Solid Edge part; units mm, degrees
sketch "Sketch1" plane through (0, 0, 0) normal (0, -1, 0) x (1, 0, 0)
  line L0 (-60, 0) -> (-60, 9)
  line L1 (-60, 9) -> (-59, 10)
  line L2 (-59, 10) -> (164, 10)
  line L3 (164, 16) -> (164, 10)
  line L4 (176, 16) -> (164, 16)
  line L5 (176, 10) -> (176, 16)
  line L6 (194, 10) -> (176, 10)
  line L7 (194, 8) -> (194, 10)
  line L8 (224, 8) -> (194, 8)
  line L9 (224, 6) -> (224, 8)
  line L10 (239, 6) -> (224, 6)
  line L11 (239, 6) -> (240, 5)
  line L12 (240, 0) -> (240, 5)
revolve "RevolvedProtrusion1" add sketch "Sketch1" angle 360 about axis through (-60, 0, 0) along (1, 0, 0)
cosmetic_thread "Thread1"
cosmetic_thread "Thread2"
sketch "Sketch2" plane through (224, 0, 0) normal (1, 0, 0) x (0, 1, 0)
  line L0 (-2.5, 5.5) -> (2.5, 5.5)
  line L1 (2.5, 5.5) -> (2.5, 10.5)
  line L2 (2.5, 10.5) -> (-2.5, 10.5)
  line L3 (-2.5, 10.5) -> (-2.5, 5.5)
extrude "Cutout1" cut sketch "Sketch2" against normal blind 30
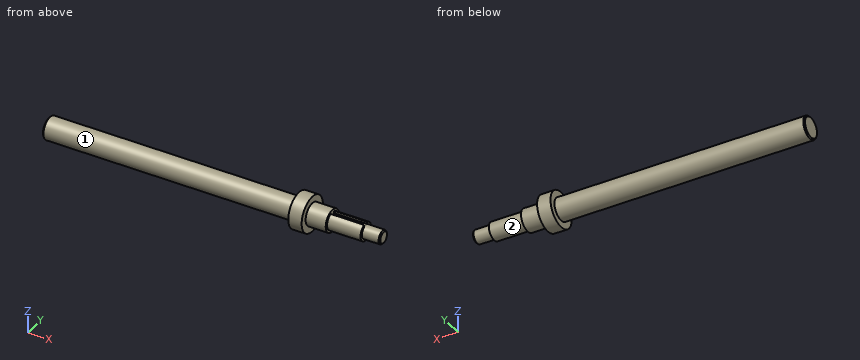
Input: part model. Units: mm. Frame: model coordinates. Face numbers are marked on the shaded views. A direction names the side the tool comes from. Round coordinates to 2 decimals unless told otherwise and drop trailing zeros. Loops run counter-clockwise (first coordinate to the right, second up) from the corner with the lowest first, then second, coordinate; pieces in that order, holes last. Notation, with made-up numbers: (14, 54) - (20, 54) arc R13 ccw to (20, 75) - close; hole circle Ø9 at (61, -1.5). An arc over 180 degrees is marked (long way). One line per item, written item: value. Start each with the question number.
(1) Section C-C, the plane z = 13. Return loops of the section in (x, y), plus the area to 3 significant figures.
(2) Section B-B, the plane x = 159. Return loops of the section in (y, z).
(3) Access query for the marked faces 1 and 2. Directions: +Z, -Z, +X, -X, +Y, -Y. A direction counts if a zero-diameter tool reaches every point of the face in a straight line with its end or side. Return the directions, or none.
(4) Contact query for flat-ended pins moving along their axis: P1, Ø5, axis at x = 183, y = 7, coming from the -Z side; P2, Ø5, axis at y = -2.5, z = -12.5, coming from the -X side; P3, Ø5, axis at x = 114.5, z = 8, coming from the -Y side. Output: stop coordinate, or through.
(5) Ray query, line 1 (X direction, y = -4, z = 14.5); line 2 (Y direction, x = 24, z = -8); line 3 (X direction, y = -2.5, z = -7.5). Return the intervals inside material, ascending. Write a range as [from, to].
(6) Section A-A, the plane z = 0. Return loops of the section in (x, y), plus the area to 3 significant figures.
Results below:
1. outline: (164, -9.33) - (176, -9.33) - (176, 9.33) - (164, 9.33) - close
1. area: 224 mm^2
2. outline: circle Ø20 at (0, 0)
3. face 1: -X
3. face 2: +X
4. P1: z = -8.93
4. P2: x = 164
4. P3: y = -8.35
5. line 1: [164, 176]
5. line 2: [-6, 6]
5. line 3: [-60, 224]
6. outline: (-60, -9) - (-59, -10) - (164, -10) - (164, -16) - (176, -16) - (176, -10) - (194, -10) - (194, -8) - (224, -8) - (224, -6) - (239, -6) - (240, -5) - (240, 5) - (239, 6) - (224, 6) - (224, 8) - (194, 8) - (194, 10) - (176, 10) - (176, 16) - (164, 16) - (164, 10) - (-59, 10) - (-60, 9) - close
6. area: 5,890 mm^2
